Input: part model. Units: mm. Frame: model coordinates. A direction names the side the tool comes from. Round coordinates to 2 decimals unless told otherwise and drop trailing zeros. Loops run counter-clockwise (first coordinate to the right, second up) from the corner with the lowest first, then second, coordinate; pieces in that order, holes last. Notation, with made-up numbers: M 50,78.5 L 81,78.5 A17 ccw 81,85.5 Z; hole C 33,9 d9. An arc over 180 degrees is marked long. Use one line per item in the form item = value. Start each with the question number.
Q1. Section query D-D, the plane y = 12. Output: boundary loops of the cut face in (x, z).
Q2. Section query A-A, the plane z = -1.75. Output: boundary loops of the cut face in (x, y), and give its area (3 significant figures).
Q3. Mould query, pull axis Z, two halves, no side actions, for faces 1 (the flat face through (30, 0, 0)), 2 (the cylindrical face through (-27.885, 31.371, 0.976)), 3 (the flat face through (5, 11, 11)), 4 (the cylindrical face through (41.827, 2.465, 0.705)). Classes: pulls with the +Z half, pulls with the -Z half, needs draft (parallel to the pull), parting line crosses it, or undercut.
Q4. First-contact query: P1, Ø6.5, axis at x = 40, z = 0, coming from the +Y side; P2, Ø13, axis at x = 11.5, z = 3, coming from the +Y side; P3, Ø12, axis at x = -25, z = -2, coming from the -Y side. Flat tips, straight axial feed; report the tip coordinate or a pass-through.
Q5. Access query for faces 5 (the cylindrical face through (-38.935, 44.305, -0.154)), 6 (the flat face through (10, 3, 0)), 7 (the flat face through (41, 5, 0)). Directions: +Z, -Z, +X, -X, +Y, -Y. A direction counts if a zero-diameter tool reaches every point of the face in a straight line with its end or side. Return the directions, or none.
Q6. Section query B-B, the plane x = 45. Output: boundary loops of the cut face in (y, z), and give its area (3 significant figures).
Q7. Ray query, line 1 along X through (y, z) = (3.9, 0) (3 decimals); line 2 along Y through (x, z) = (-9, 9); line 3 along X through (y, z) = (3.25, 0). Return the intervals inside material, ascending.
Q8. Section query C-C, the plane z = 4.75. Output: boundary loops of the cut face in (x, y).
```python
from build123d import *

# Parameters (mm, degrees)
EXTRUDE_1_DEPTH     = 11
SKETCH_2_R          = 3.25
CUT_EXTRUDE_1_DEPTH = 5
SKETCH_3_R          = 3.25
CUT_EXTRUDE_2_DEPTH = 5
FILLET_1_R          = 4
FILLET_2_R          = 1


with BuildPart() as part:
    # Эскиз1 → Бобышка-Вытянуть1 (new body, symmetric)
    with BuildSketch(Plane.XY):
        Polygon((0, 0), (-42.426406871, 42.426406871), (-38.890872965, 45.961940777), (-15.028558569, 22.099626381), (26.253591352, 5), (60, 5), (60, 0), align=None)
        Polygon((-14.313708499, 18.556349186), (23.242640687, 3), (1.242640687, 3), align=None, mode=Mode.SUBTRACT)
    extrude(amount=EXTRUDE_1_DEPTH, both=True)

    # Эскиз2 → Вырез-Вытянуть1 (cut)
    with BuildSketch(Plane(origin=(0, 0, 0), x_dir=(0, 0, 1), z_dir=(-0.707106781, -0.707106781, 0))):
        with Locations(Location((0, 45, 0), (0, 0, 270))):  # turned: the seam where the file's is
            Circle(SKETCH_2_R)
    extrude(amount=-CUT_EXTRUDE_1_DEPTH, mode=Mode.SUBTRACT)

    # Эскиз3 → Вырез-Вытянуть2 (cut)
    with BuildSketch(Plane.XZ):
        with Locations(Location((45, 0, 0), (0, 0, 270))):  # turned: the seam where the file's is
            Circle(SKETCH_3_R)
    extrude(amount=-CUT_EXTRUDE_2_DEPTH, mode=Mode.SUBTRACT)

    # Скругление1
    fillet_1_edges = [part.edges().sort_by_distance(p)[0] for p in [
        (-38.890872965, 45.961940777, 0),
        (60, 5, 0),
    ]]
    fillet(fillet_1_edges, radius=FILLET_1_R)

    # Скругление2
    fillet_2_edges = [part.edges().sort_by_distance(p)[0] for p in [
        (-14.313708499, 18.556349186, 0),
        (1.242640687, 3, 0),
        (23.242640687, 3, 0),
    ]]
    fillet(fillet_2_edges, radius=FILLET_2_R)


solid = part.part
```
Results found:
q1.outline = M -12,-11 L -7.76,-11 L -7.76,11 L -12,11 Z; M 1.51,-11 L 9.35,-11 L 9.35,11 L 1.51,11 Z
q2.outline = M -42.43,42.43 L -33.76,33.76 L -30.22,37.29 L -36.06,43.13 A4 ccw -41.72,43.13 Z; M -29.88,29.88 L 0,0 L 42.26,0 L 42.26,5 L 26.25,5 L -15.03,22.1 L -26.35,33.42 Z; M 47.74,0 L 60,0 L 60,1 A4 ccw 56,5 L 47.74,5 Z; hole M -10.76,15 L 0.95,3.29 A1 ccw 1.66,3 L 18.22,3 A1 ccw 18.6,4.92 L -9.67,16.63 A1 ccw Z
q2.area = 571 mm²
q3.face_1 = needs draft
q3.face_2 = undercut
q3.face_3 = pulls with the +Z half
q3.face_4 = undercut
q4.P1 = 5
q4.P2 = 13.8
q4.P3 = 19
q5.face_5 = +Z, -Z, +Y
q5.face_6 = +Z, -Z
q5.face_7 = +Z, -Z, +X, +Y
q6.outline = M 0,-11 L 5,-11 L 5,-3.25 L 0,-3.25 Z; M 0,3.25 L 5,3.25 L 5,11 L 0,11 Z
q6.area = 77.5 mm²
q7.line_1 = -3.9 to 0.343, 19.21 to 41.75, 48.25 to 58.755
q7.line_2 = 9 to 13.24, 16.36 to 19.6
q7.line_3 = -3.25 to 1, 18.88 to 41.75, 48.25 to 59.31
q8.outline = M -42.43,42.43 L 0,0 L 60,0 L 60,1 A4 ccw 56,5 L 26.25,5 L -15.03,22.1 L -36.06,43.13 A4 ccw -41.72,43.13 Z; hole M -10.76,15 L 0.95,3.29 A1 ccw 1.66,3 L 18.22,3 A1 ccw 18.6,4.92 L -9.67,16.63 A1 ccw Z
